Build history of the part. All positions in model axes, mm. Face numbers are marked on the shaded views. A direction names the side the tool comes from. Give positions to 0.01 mm unless a question says otherwise; leave off trailing zeros. Loops run counter-clockwise (first coordinate to the right, second up) from the corner with the lowest first, then second, coordinate; pieces in that order, holes last. Notation, with made-up numbers: (36, 80) -> (86, 80) arc R28 ccw to (86, 109) -> close; hole circle Ø10 at (-26.5, 63.5). An arc over 180 degrees is marked (long way). Answer as a JSON object with one key per item and string values. Group by question number.
Q1. Band-saw the part on B-B, the plane y = 0. Write the cut outline in (x, z).
Q2. Two-plate mould, pull along X, no slides. Class the marked faces 4, 5 and 6: pulls with the +X half, pulls with the -X half, needs draft (parallel to the pull), parting line crosses it, or undercut.
Q3. Wall check: probe 1 along Z at (x, y) = (-9.8, 0); probe 2 along X at (y, z) = (3.5, 0.5); probe 3 along Z at (x, y) = (-2, -4). Give the ranges that are in metal, low to high. Write a range as from..to.
Q4. Tool access for the marked faces 1, 2 and 3: list every direction of +Z, -Z, +X, -X, +Y, -Y with a clear straight run to the whole face (end or side of a thin tool).
Q5. Band-saw the part on A-A, the plane z = 15. Write the cut outline in (x, y).
Q6. Band-saw the part on D-D, the plane z = 2.5. Write the cut outline in (x, y), plus the area to 3 significant figures.
Q7. Drop flat-ended pins along their axis: pin 1 (1.5 mm diameter, centred on x = -4.5, y = -2, fed in from -Z); pin 2 (2.5 mm diameter, centred on x = 2, z = 10.5, fed in from -Y); pin 3 (2.5 mm diameter, centred on y = 0, z = 15, fed in from -X); pin 4 (2 mm diameter, centred on x = 5, z = 10.5, fed in from +Y). Give the stop position or say it passes through.
Q8. Band-saw the part on C-C, the plane x = 5. Write the cut outline in (y, z), plus the area to 3 significant figures.
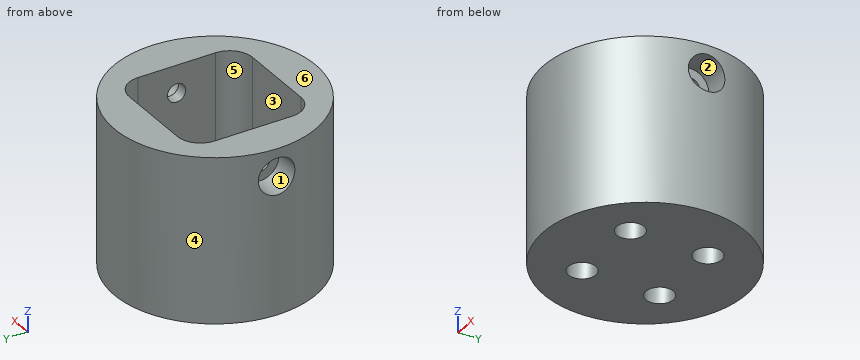
from build123d import *

# Parameters (mm, degrees)
SKETCH1_R               = 11
SKETCH1_R_2             = 1.5
BOSS_EXTRUDE1_DEPTH     = 18
CUT_EXTRUDE2_DEPTH      = 24.790754507
CUT_EXTRUDE2_DEPTH_BACK = 24.790754507
SKETCH3_R               = 1
CUT_EXTRUDE3_START      = -8
SKETCH4_R               = 2
CUT_EXTRUDE3_DEPTH      = 5
CUT_EXTRUDE4_START      = 13
SKETCH4_2_R             = 2
CUT_EXTRUDE4_DEPTH      = 5
CUT_EXTRUDE5_START      = -16
SKETCH2_R               = 2.5
SKETCH2_R_2             = 1.5
CUT_EXTRUDE5_DEPTH      = 16


with BuildPart() as part:
    # Sketch1 → Boss-Extrude1 (new body)
    with BuildSketch(Plane.XY):
        Circle(SKETCH1_R)
        with Locations((-4.242640687, 4.242640687)):
            Circle(SKETCH1_R_2, mode=Mode.SUBTRACT)
        with Locations((4.242640687, 4.242640687)):
            Circle(SKETCH1_R_2, mode=Mode.SUBTRACT)
        with Locations((4.242640687, -4.242640687)):
            Circle(SKETCH1_R_2, mode=Mode.SUBTRACT)
        with Locations((-4.242640687, -4.242640687)):
            Circle(SKETCH1_R_2, mode=Mode.SUBTRACT)
    extrude(amount=BOSS_EXTRUDE1_DEPTH)

    # Sketch3 → Cut-Extrude2 (cut, two sides: drawn at the far end of the back side and taken through both)
    with BuildSketch(Plane(origin=(0, 0, 0), x_dir=(0, 0, -1), z_dir=(1, 0, 0)).offset(-CUT_EXTRUDE2_DEPTH_BACK)):
        with Locations((-15, 0)):
            Circle(SKETCH3_R)
    extrude(amount=CUT_EXTRUDE2_DEPTH + CUT_EXTRUDE2_DEPTH_BACK, mode=Mode.SUBTRACT)

    # Sketch4 → Cut-Extrude3 (cut)
    with BuildSketch(Plane(origin=(0, 0, 0), x_dir=(0, 0, -1), z_dir=(1, 0, 0)).offset(CUT_EXTRUDE3_START)):
        with Locations((-15, 0)):
            Circle(SKETCH4_R)
    extrude(amount=-CUT_EXTRUDE3_DEPTH, mode=Mode.SUBTRACT)

    # Sketch4_2 → Cut-Extrude4 (cut)
    with BuildSketch(Plane(origin=(0, 0, 0), x_dir=(0, 0, -1), z_dir=(1, 0, 0)).offset(CUT_EXTRUDE4_START)):
        with Locations((-15, 0)):
            Circle(SKETCH4_2_R)
    extrude(amount=-CUT_EXTRUDE4_DEPTH, mode=Mode.SUBTRACT)

    # Sketch2 → Cut-Extrude5 (cut)
    # profile 1 of 9: a face of its own
    with BuildSketch(Plane.XY.offset(18).offset(CUT_EXTRUDE5_START)):
        with BuildLine():
            Line((4.242640687, 6.742640687), (-4.242640687, 6.742640687))
            ThreePointArc((-4.242640687, 6.742640687), (-2.474873734, 6.01040764), (-1.742640687, 4.242640687))
            ThreePointArc((-1.742640687, 4.242640687), (-4.242640687, 1.742640687), (-6.742640687, 4.242640687))
            Line((-6.742640687, 4.242640687), (-6.742640687, -4.242640687))
            ThreePointArc((-6.742640687, -4.242640687), (-4.242640687, -1.742640687), (-1.742640687, -4.242640687))
            ThreePointArc((-1.742640687, -4.242640687), (-2.474873734, -6.01040764), (-4.242640687, -6.742640687))
            Line((-4.242640687, -6.742640687), (4.242640687, -6.742640687))
            ThreePointArc((4.242640687, -6.742640687), (2.474873734, -2.474873734), (6.742640687, -4.242640687))
            Line((6.742640687, -4.242640687), (6.742640687, 4.242640687))
            ThreePointArc((6.742640687, 4.242640687), (2.474873734, 2.474873734), (4.242640687, 6.742640687))
        make_face()
    # profile 2 of 9: a face of its own
    with BuildSketch(Plane.XY.offset(18).offset(CUT_EXTRUDE5_START)):
        with Locations((4.242640687, 4.242640687)):
            Circle(SKETCH2_R)
        with Locations((4.242640687, 4.242640687)):
            Circle(SKETCH2_R_2, mode=Mode.SUBTRACT)
    # profile 3 of 9: a face of its own
    with BuildSketch(Plane.XY.offset(18).offset(CUT_EXTRUDE5_START)):
        with Locations((-4.242640687, 4.242640687)):
            Circle(SKETCH2_R)
        with Locations((-4.242640687, 4.242640687)):
            Circle(SKETCH2_R_2, mode=Mode.SUBTRACT)
    # profile 4 of 9: a face of its own
    with BuildSketch(Plane.XY.offset(18).offset(CUT_EXTRUDE5_START)):
        with Locations((-4.242640687, 4.242640687)):
            Circle(SKETCH2_R_2)
    # profile 5 of 9: a face of its own
    with BuildSketch(Plane.XY.offset(18).offset(CUT_EXTRUDE5_START)):
        with Locations((-4.242640687, -4.242640687)):
            Circle(SKETCH2_R)
        with Locations((-4.242640687, -4.242640687)):
            Circle(SKETCH2_R_2, mode=Mode.SUBTRACT)
    # profile 6 of 9: a face of its own
    with BuildSketch(Plane.XY.offset(18).offset(CUT_EXTRUDE5_START)):
        with Locations((-4.242640687, -4.242640687)):
            Circle(SKETCH2_R_2)
    # profile 7 of 9: a face of its own
    with BuildSketch(Plane.XY.offset(18).offset(CUT_EXTRUDE5_START)):
        with Locations((4.242640687, -4.242640687)):
            Circle(SKETCH2_R)
        with Locations((4.242640687, -4.242640687)):
            Circle(SKETCH2_R_2, mode=Mode.SUBTRACT)
    # profile 8 of 9: a face of its own
    with BuildSketch(Plane.XY.offset(18).offset(CUT_EXTRUDE5_START)):
        with Locations((4.242640687, -4.242640687)):
            Circle(SKETCH2_R_2)
    # profile 9 of 9: a face of its own
    with BuildSketch(Plane.XY.offset(18).offset(CUT_EXTRUDE5_START)):
        with Locations((4.242640687, 4.242640687)):
            Circle(SKETCH2_R_2)
    extrude(amount=CUT_EXTRUDE5_DEPTH, mode=Mode.SUBTRACT)


solid = part.part
Worked answers:
{
 "1": {"outline": "(-11, 0) -> (11, 0) -> (11, 13) -> (8, 13) -> (8, 14) -> (6.74, 14) -> (6.74, 2) -> (-6.74, 2) -> (-6.74, 14) -> (-8, 14) -> (-8, 13) -> (-11, 13) -> close; (-11, 17) -> (-8, 17) -> (-8, 16) -> (-6.74, 16) -> (-6.74, 18) -> (-11, 18) -> close; (6.74, 16) -> (8, 16) -> (8, 17) -> (11, 17) -> (11, 18) -> (6.74, 18) -> close"},
 "2": {"face 4": "parting line crosses it", "face 5": "undercut", "face 6": "needs draft"},
 "3": {"probe 1": "0..13, 17..18", "probe 2": "-10.43..-5.55, -2.94..2.94, 5.55..10.43", "probe 3": "0..2"},
 "4": {"face 1": "-X", "face 2": "+X", "face 3": "+Z"},
 "5": {"outline": "(-10.82, -2) arc R11 ccw to (10.82, -2) -> (8, -2) -> (8, -1) -> (6.74, -1) -> (6.74, -4.24) arc R2.5 cw to (4.24, -6.74) -> (-4.24, -6.74) arc R2.5 cw to (-6.74, -4.24) -> (-6.74, -1) -> (-8, -1) -> (-8, -2) -> close; (-10.82, 2) -> (-8, 2) -> (-8, 1) -> (-6.74, 1) -> (-6.74, 4.24) arc R2.5 cw to (-4.24, 6.74) -> (4.24, 6.74) arc R2.5 cw to (6.74, 4.24) -> (6.74, 1) -> (8, 1) -> (8, 2) -> (10.82, 2) arc R11 ccw to start"},
 "6": {"outline": "circle Ø22 at (0, 0); hole (-6.74, -4.24) arc R2.5 ccw to (-4.24, -6.74) -> (4.24, -6.74) arc R2.5 ccw to (6.74, -4.24) -> (6.74, 4.24) arc R2.5 ccw to (4.24, 6.74) -> (-4.24, 6.74) arc R2.5 ccw to (-6.74, 4.24) -> close", "area": "204 mm2"},
 "7": {"pin 1": "z = 0", "pin 2": "y = -10.97", "pin 3": "x = -8", "pin 4": "y = 10.25"},
 "8": {"outline": "(-9.8, 0) -> (-5.54, 0) -> (-5.54, 2) -> (-6.63, 2) -> (-6.63, 18) -> (-9.8, 18) -> close; (-2.95, 0) -> (2.95, 0) -> (2.95, 2) -> (-2.95, 2) -> close; (5.54, 0) -> (9.8, 0) -> (9.8, 18) -> (6.63, 18) -> (6.63, 2) -> (5.54, 2) -> close", "area": "130 mm2"}
}
